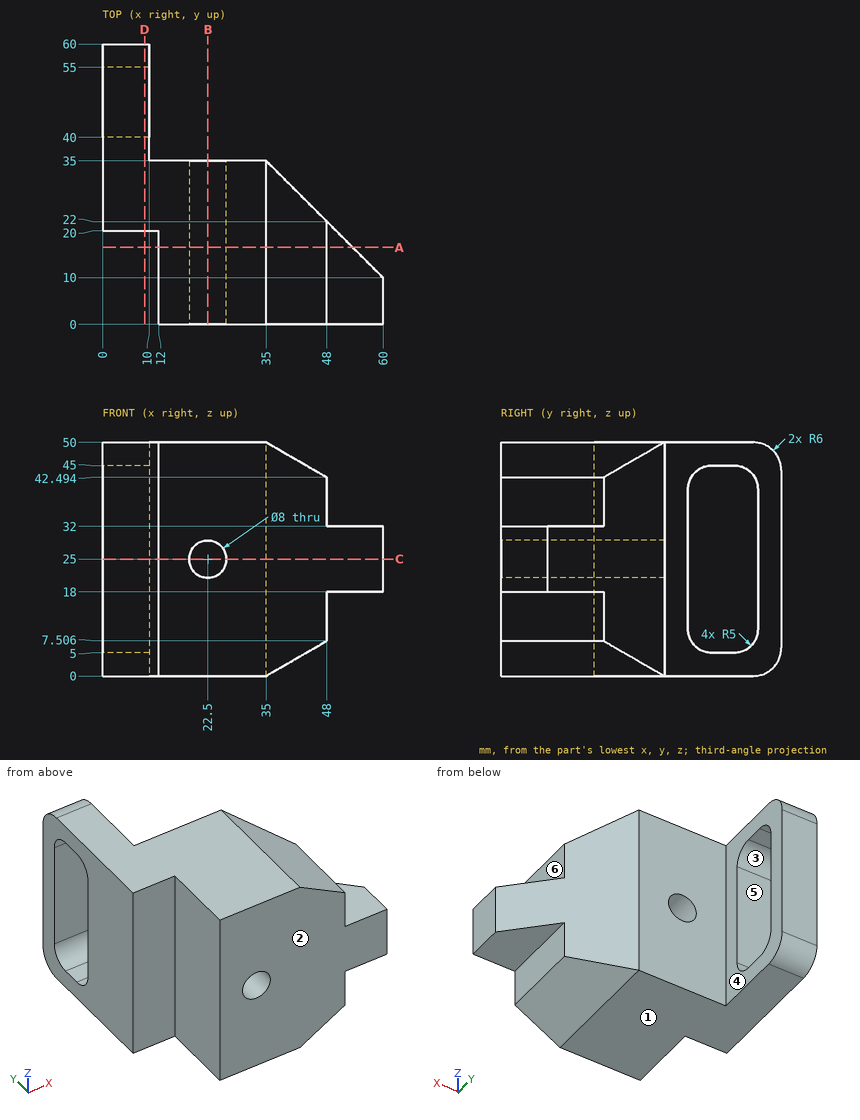
Geometry check sheet. Reference: drawing and pictorial views, mm from the part's lowest x, y, z. A direction names the side the tool comes from. Coordinates: 2 decimals unless noted, no trailing zeros. Loops run counter-clockwise (first coordinate to the right, second up) from the corner with the lowest first, then second, coordinate; pieces in that order, holes last. Notation, with made-up numbers: (-11.75, 41) -> (28.25, 41) arc R31 cw to (28.25, 75) -> close; hole circle Ø10 at (65.5, 43.5). An arc over 180 degrees is marked (long way). Write item = value, one per line. Start each with the question number.
1. Section check A-A on y = 16.5. Record the cut outline in (x, z) (1 decimal), then the cut area to 3 significant figures.
2. Tool access check on the marked faces 4, 5 and 6. Record the directions out of +Z, -Z, +X, -X, +Y, -Y that give a thin tool (end or side, any length) a straight path to the whole face; none if there is none.
3. Section check C-C on z = 25. Record the cut outline in (x, y).
4. Section check B-B on x = 22.5. Record the cut outline in (y, z), then the cut area to 3 significant figures.
5. Draft check along Z on the marked faces 1, 2 and 3. Enter one of: released by +Z, released by -Z, zero draft, split by the parting line, or undercut.
6. Depth check by flat-ended pin: P1, Ø5, axis at y = 11.5, z = 14, coming from the +X side; P2, Ø3.5, axis at x = 5.5, z = 20, coming from the -Y side; P3, Ø9.5, axis at x = 51.5, y = 11, coming from the +Z side (1 decimal); P4, Ø6.5, axis at x = 22.5, z = 25, coming from the +Y side. Enter the tip coordinate at first touch or a pass-through.
7. Section check D-D on x = 9. Record the cut outline in (y, z), then the cut area to 3 significant figures.
8. Material ranges on line 1 (Y direction, x = 7, z = 32); line 2 (X direction, y = 15, z = 25); line 3 (Z direction, x = 22.5, y = 25), recorded low to high.
Responses:
q1.outline = (12, 0) -> (35, 0) -> (48, 7.5) -> (48, 18) -> (53.5, 18) -> (53.5, 32) -> (48, 32) -> (48, 42.5) -> (35, 50) -> (12, 50) -> close; hole circle Ø8 at (22.5, 25)
q1.area = 1,730 mm2
q2.face_4 = +Z, -Z, +X, +Y
q2.face_5 = +X, -X
q2.face_6 = +Z, +X, +Y, -Y
q3.outline = (0, 20) -> (12, 20) -> (12, 0) -> (18.5, 0) -> (18.5, 35) -> (10, 35) -> (10, 40) -> (0, 40) -> close; (0, 55) -> (10, 55) -> (10, 60) -> (0, 60) -> close; (26.5, 0) -> (60, 0) -> (60, 10) -> (35, 35) -> (26.5, 35) -> close
q4.outline = (0, 0) -> (35, 0) -> (35, 21) -> (0, 21) -> close; (0, 29) -> (35, 29) -> (35, 50) -> (0, 50) -> close
q4.area = 1,470 mm2
q5.face_1 = released by -Z
q5.face_2 = zero draft
q5.face_3 = undercut
q6.P1 = 48
q6.P2 = 20
q6.P3 = 43.2
q6.P4 = through
q7.outline = (20, 0) -> (54, 0) arc R6 ccw to (60, 6) -> (60, 44) arc R6 ccw to (54, 50) -> (20, 50) -> close; hole (40, 10) arc R5 ccw to (45, 5) -> (50, 5) arc R5 ccw to (55, 10) -> (55, 40) arc R5 ccw to (50, 45) -> (45, 45) arc R5 ccw to (40, 40) -> close
q7.area = 1,410 mm2
q8.line_1 = 20 to 40, 55 to 60
q8.line_2 = 12 to 18.5, 26.5 to 55
q8.line_3 = 0 to 21, 29 to 50
